Geometry: final body of the model. Coordinates: model frame, mm. Give positions to 0.01 mm unless a question says otherwise; leave off trailing zeros. Loops run counter-clockwise (first coordinate to the right, second up) from the corner with the lowest first, then second, coordinate; pieces in that order, holes last. Notation, with made-up numbers: (5.5, -34.75) -> (15.5, -34.75) arc R26 ccw to (15.5, -6.75) -> close; hole circle Ø6 at (22.25, 19). An arc over 180 degrees is marked (long way). One line per question, with ' | ' between items. Start each with the question number.
Item 1: Section C-C on z = 0. Return loops of the section in (x, y) (3 decimals), then the cut area to 3 significant figures.
Item 2: Section B-B on x = 145. Return loops of the section in (y, z) (3 decimals), then the cut area to 3 significant figures.
Item 3: Section D-D on x = 95. Return loops of the section in (y, z) (3 decimals).
Item 4: Pin query (flat end, axial travel): P1, Ø5, axis at x = 20, z = -18.75, coming from the -Y side; P2, Ø1.5, axis at y = 0.5, z = 18.5, coming from the -X side. Return the tip coordinate at first contact, or that it passes through.
Item 5: Material intervals for line 1 along Z through (x, y) = (20, 2.35); line 2 along Z through (x, y) = (-16.25, 2.15); line 3 along X through (y, z) = (1.8, -18.75), sorted ascending. Write a range as [from, to].
Item 6: Section A-A on y = 2.05. Give the number of separate pieces and of enclosed holes in the cut face, then the cut area to 3 significant figures.
Item 7: Mould query, pull axis Z, two halves, no side actions, for faces 1 (the cylindrical face through (0.54, 1.57, 2.44)), 2 (the cylindrical face through (-22.15, 1.61, -24.49)), 3 (the cylindrical face through (-22.15, 1.61, 24.49)). Classes: released by +Z, released by -Z, zero draft, split by the parting line, or undercut.
from build123d import *

# Parameters (mm, degrees)
SKETCH1_W             = 195
SKETCH1_H             = 55
BOSS_EXTRUDE1_DEPTH   = 3.175
FILLET1_R             = 10
F_5_0MM_DOWEL_HOLE1_D = 5
F_4_0MM_DOWEL_HOLE1_D = 4
F_5_0MM_DOWEL_HOLE2_D = 5


with BuildPart() as part:
    # Sketch1 → Boss-Extrude1 (new body)
    with BuildSketch(Plane(origin=(0, 0, 0), x_dir=(1, 0, 0), z_dir=(0, 1, 0))):
        with Locations((72.5, 0)):
            Rectangle(SKETCH1_W, SKETCH1_H)
    extrude(amount=BOSS_EXTRUDE1_DEPTH)

    # Fillet1
    fillet1_edges = [part.edges().sort_by_distance(p)[0] for p in [
        (-25, 1.5875, -27.5),
        (170, 1.5875, -27.5),
        (170, 1.5875, 27.5),
        (-25, 1.5875, 27.5),
    ]]
    fillet(fillet1_edges, radius=FILLET1_R)

    # Ø5.0mm Dowel Hole1 (through all)
    with Locations(Plane(origin=(0, 3.175, 0), x_dir=(1, 0, 0), z_dir=(0, 1, 0))):
        with Locations((0, 0)):
            Hole(F_5_0MM_DOWEL_HOLE1_D / 2)

    # Ø4.0mm Dowel Hole1 (through all)
    with Locations(Plane(origin=(0, 3.175, 0), x_dir=(1, 0, 0), z_dir=(0, 1, 0))):
        with Locations((-16.25, -18.75), (20, -18.75), (95, -18.75), (95, 18.75), (20, 18.75), (-16.25, 18.75)):
            Hole(F_4_0MM_DOWEL_HOLE1_D / 2)

    # Ø5.0mm Dowel Hole2 (through all)
    with Locations(Plane(origin=(0, 3.175, 0), x_dir=(1, 0, 0), z_dir=(0, 1, 0))):
        with Locations((165, 20.5), (145, 20.5), (165, -20.5), (145, -20.5)):
            Hole(F_5_0MM_DOWEL_HOLE2_D / 2)


solid = part.part
Result sheet:
1) outline: (-25, 0) -> (-2.5, 0) -> (-2.5, 3.175) -> (-25, 3.175) -> close; (2.5, 0) -> (170, 0) -> (170, 3.175) -> (2.5, 3.175) -> close | area: 603 mm²
2) outline: (0, -27.5) -> (3.175, -27.5) -> (3.175, -23) -> (0, -23) -> close; (0, -18) -> (3.175, -18) -> (3.175, 18) -> (0, 18) -> close; (0, 23) -> (3.175, 23) -> (3.175, 27.5) -> (0, 27.5) -> close | area: 143 mm²
3) outline: (0, -27.5) -> (3.175, -27.5) -> (3.175, -20.75) -> (0, -20.75) -> close; (0, -16.75) -> (3.175, -16.75) -> (3.175, 16.75) -> (0, 16.75) -> close; (0, 20.75) -> (3.175, 20.75) -> (3.175, 27.5) -> (0, 27.5) -> close
4) P1: stops at y = 0 | P2: stops at x = -25
5) line 1: z = [-27.5, -20.75], [-16.75, 16.75], [20.75, 27.5] | line 2: z = [-27.42, -20.75], [-16.75, 16.75], [20.75, 27.42] | line 3: x = [-24.92, -18.25], [-14.25, 18], [22, 93], [97, 143.21], [146.79, 163.21], [166.79, 169.92]
6) separate pieces: 1 | enclosed holes: 11 | area: 10,500 mm²
7) face 1: undercut | face 2: released by -Z | face 3: released by +Z
